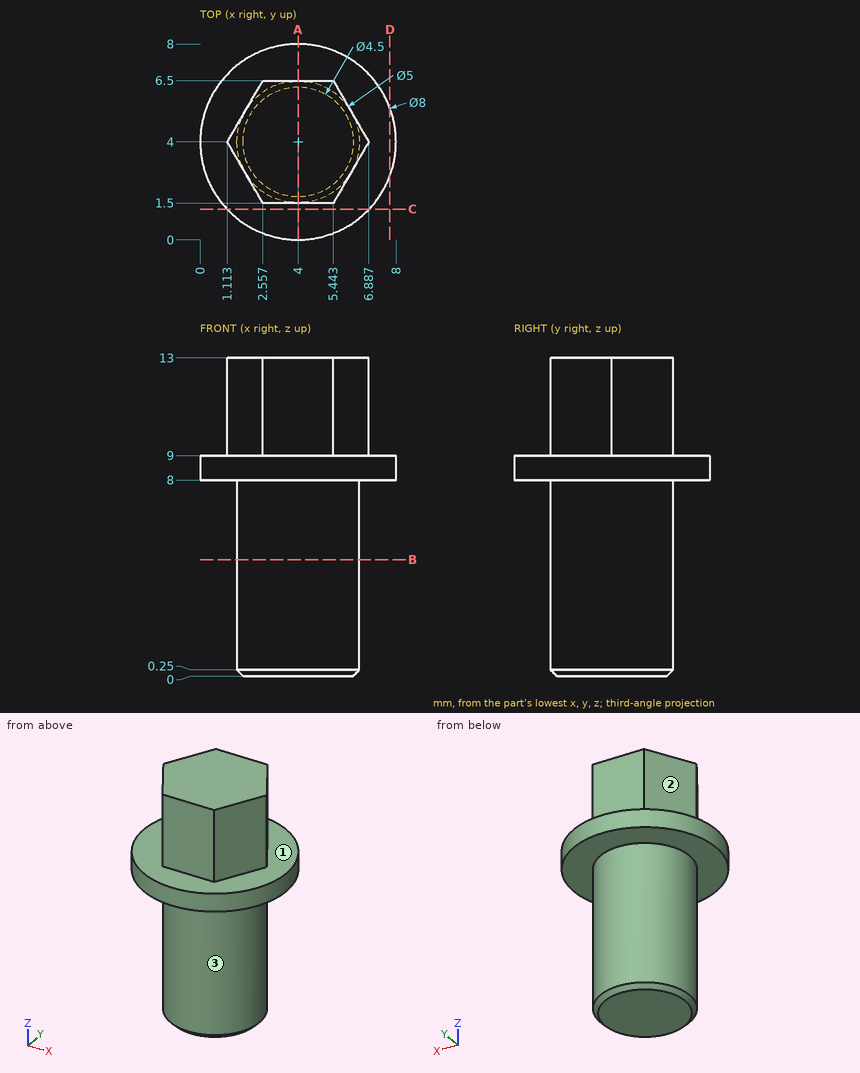
Can you work these out from the drawing? Everything is in mm from the part's minimum corner. A direction names the side the tool comes from. Round coordinates to 2 decimals unless told otherwise and drop trailing zeros. Loops run counter-clockwise (first coordinate to the right, second up) from the corner with the lowest first, then second, coordinate; pieces in that order, holes last. Notation, with made-up numbers: (-24, 86) -> (-4, 86) arc R20 cw to (-4, 91) -> close; hole circle Ø9 at (7.5, 3.5). An arc over 180 degrees is marked (long way). Answer in a Markdown table with one row per item.
Item 1: Suppose I cut it at B-B, the plane z = 4.75. List the corners of the cut face in (x, y) for me.
Answer block:
| item | result |
|---|---|
| outline | circle Ø5 at (4, 4) |
Item 2: Suppose I cut it at C-C, the plane y = 1.25. List the corners of the cut face in (x, z) for me (1 decimal).
Answer block:
| item | result |
|---|---|
| outline | (1.1, 8) -> (6.9, 8) -> (6.9, 9) -> (1.1, 9) -> close |
Item 3: On a 3-axis mill with a long thin cutter (end or side, diameter ignored), from which of +Z, -Z, +X, -X, +Y, -Y can I reach the whole of each face in a straight line? I mean the marked faces 1, 2 and 3. Say none if no direction works.
Answer block:
| item | result |
|---|---|
| face 1 | +Z |
| face 2 | +Z, -X, +Y |
| face 3 | -Z |
Item 4: If I drill on probe 1 along Z at (x, y) = (7, 6); probe 2 along Y at (x, z) = (4.25, 12.75); probe 3 along Y at (x, z) = (4.5, 6), over which ranges is the centre line in solid material (lowest first)?
Answer block:
| item | result |
|---|---|
| probe 1 | 8 to 9 |
| probe 2 | 1.5 to 6.5 |
| probe 3 | 1.55 to 6.45 |
Item 5: Suppose I cut it at D-D, the plane x = 7.75. List the corners of the cut face in (y, z) for me.
Answer block:
| item | result |
|---|---|
| outline | (2.61, 8) -> (5.39, 8) -> (5.39, 9) -> (2.61, 9) -> close |
Item 6: Suppose I cut it at A-A, the plane x = 4. List the corners of the cut face in (y, z) for me.
Answer block:
| item | result |
|---|---|
| outline | (0, 8) -> (1.5, 8) -> (1.5, 0.25) -> (1.75, 0) -> (6.25, 0) -> (6.5, 0.25) -> (6.5, 8) -> (8, 8) -> (8, 9) -> (6.5, 9) -> (6.5, 13) -> (1.5, 13) -> (1.5, 9) -> (0, 9) -> close |
Item 7: Will these pins go through, and if not, where does the flat tip stop? P1, Ø2, axis at y = 1.5, z = 6, coming from the +X side; P2, Ø0.9, axis at x = 3.5, z = 11, coming from the -Y side; P3, Ø1.5, axis at x = 2, z = 11, coming from the +Y side.
Answer block:
| item | result |
|---|---|
| P1 | x = 6 |
| P2 | y = 1.5 |
| P3 | y = 6.5 |
